Geometry: see drawing. Coordinates: mm, zero at the bounding-box minimum. A direction names the side the tool comes from. Give positions to 0.01 mm unless a question says otherwise; leave off trailing zeros. Loops run counter-clockwise (first coordinate to the right, second up) from the corner with the lowest first, then second, coordinate; pieces in that order, holes last. Notation, with made-up numbers: M -33.5,40 L 8.5,40 A26 ccw 8.5,76 Z; hole C -40,-0.75 d2. An arc over 180 degrees is marked long. Use a Markdown table: item, result. Add a question column.
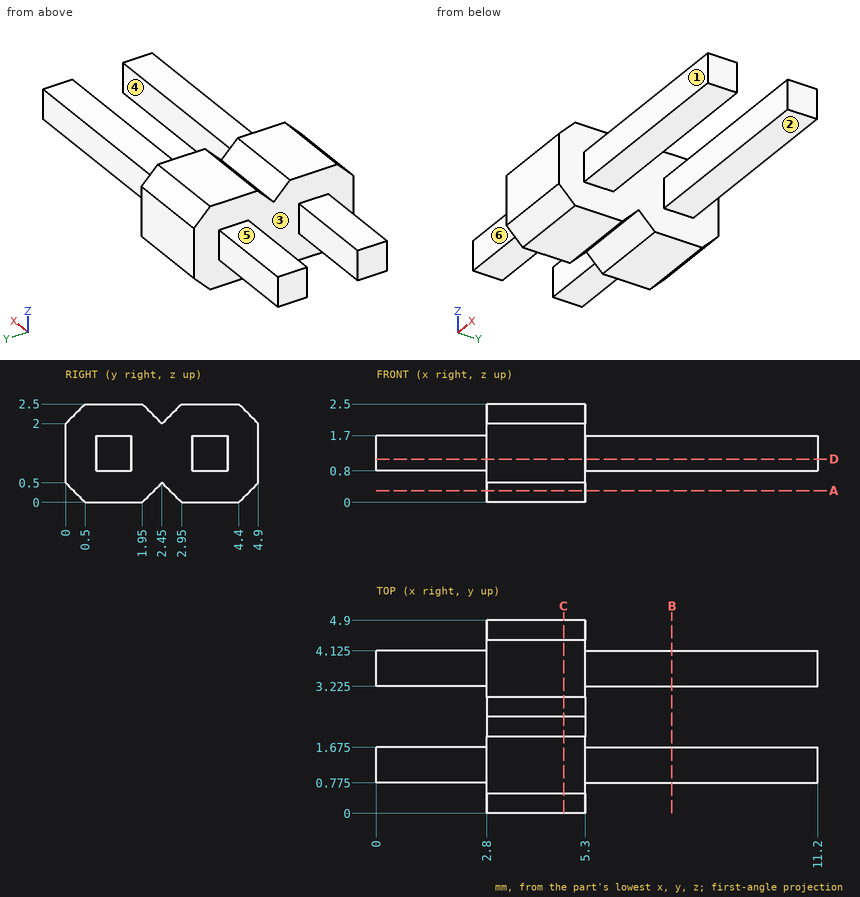
1) Contact query for flat-ended pins moving along their axis: P1, Ø1, axis at x = 8.5, z = 2, coming from the -Y side (3 decimals); P2, Ø0.7, axis at x = 9.5, z = 1, coming from the +Y side (3 decimals); P3, Ø0.5, axis at x = 1, y = 3.5, coming from the +Z side. Output: stop coordinate, or through.
2) Section query D-D, the plane z = 1.1. Return the cut outline in (x, y) (3 decimals), and give its area (3 significant figures).
3) Ray query, line 1 (Y direction, x = 7.75, z = 1.25) (3 decimals); line 2 (X direction, y = 3.1, z = 0.8); line 3 (Z direction, x = 4.5, y = 0.35). Return the intervals inside material, ascending. Write a range as [from, to].
4) Section query C-C, the plane x = 4.75. Return the cut outline in (y, z), and give its area (4 significant figures).
5) Reachability of the marked faces 4, 5 and 6 from +Z, -Z, +X, -X, +Y, -Y: full face, straight path, thin tool, end or side. Return the list, or none.
6) Pull-direction query (Y, two-part tool) for the marked faces 1, 2 and 3; classes: pulls with the +Y half, pulls with the -Y half, needs draft (parallel to the pull), parting line crosses it, or undercut.
7) Section query A-A, the plane z = 0.3. Return the cut outline in (x, y).
8) Section query B-B, the plane x = 7.5. Return the cut outline in (y, z) (3 decimals).
Entries:
| question | item | result |
|---|---|---|
| 1 | P1 | stops at y = 0.775 |
| 1 | P2 | stops at y = 4.125 |
| 1 | P3 | stops at z = 1.7 |
| 2 | outline | M 0,0.775 L 2.8,0.775 L 2.8,0 L 5.3,0 L 5.3,0.775 L 11.2,0.775 L 11.2,1.675 L 5.3,1.675 L 5.3,3.225 L 11.2,3.225 L 11.2,4.125 L 5.3,4.125 L 5.3,4.9 L 2.8,4.9 L 2.8,4.125 L 0,4.125 L 0,3.225 L 2.8,3.225 L 2.8,1.675 L 0,1.675 Z |
| 2 | area | 27.9 mm² |
| 3 | line 1 | y = [0.775, 1.675], [3.225, 4.125] |
| 3 | line 2 | x = [2.8, 5.3] |
| 3 | line 3 | z = [0.15, 2.35] |
| 4 | outline | M 0,0.5 L 0.5,0 L 1.95,0 L 2.45,0.5 L 2.95,0 L 4.4,0 L 4.9,0.5 L 4.9,2 L 4.4,2.5 L 2.95,2.5 L 2.45,2 L 1.95,2.5 L 0.5,2.5 L 0,2 Z |
| 4 | area | 11.25 mm² |
| 5 | face 4 | +Z, -Z, +X |
| 5 | face 5 | +Z, -X, +Y, -Y |
| 5 | face 6 | +Z, -Z, -X, -Y |
| 6 | face 1 | pulls with the -Y half |
| 6 | face 2 | needs draft |
| 6 | face 3 | undercut |
| 7 | outline | M 2.8,0.2 L 5.3,0.2 L 5.3,2.25 L 2.8,2.25 Z; M 2.8,2.65 L 5.3,2.65 L 5.3,4.7 L 2.8,4.7 Z |
| 8 | outline | M 0.775,0.8 L 1.675,0.8 L 1.675,1.7 L 0.775,1.7 Z; M 3.225,0.8 L 4.125,0.8 L 4.125,1.7 L 3.225,1.7 Z |
